Verification items for the finished model (mm, model axes). A direction names the side the tool comes from. Coordinates: 2 decimals unless noted, no trailing zeros. Loops run counter-clockwise (first coordinate to the right, second up) from the corner with the lowest first, then second, coordinate; pieces in that order, holes last. Notation, with made-up numbers: (8.5, -12.5) -> (32.5, -12.5) arc R6 cw to (32.5, -4.5) -> close; hole circle Ø11 at (69.5, -21.5). An arc over 180 degrees is marked (long way). Use CSV: the item, a comma, the result in double quotes. Start each with the question number.
```python
from build123d import *

# Parameters (mm, degrees)
F0_W     = 10
F0_H     = 10
F1_DEPTH = 5


with BuildPart() as f1:
    # F0 (on Top) → F1 (new body)
    with BuildSketch(Plane.XY):
        with BuildLine():
            Line((-217.772444, 298.14717), (-218.393043, 298.14717))
            Line((-218.393043, 298.14717), (-218.393043, 218.14717))
            Line((-218.393043, 218.14717), (-213.393043, 218.14717))
            Line((-213.393043, 218.14717), (-213.393043, 208.14717))
            Line((-213.393043, 208.14717), (-218.393043, 208.14717))
            Line((-218.393043, 208.14717), (-218.393043, 129.632429))
            ThreePointArc((-218.393043, 129.632429), (-108.393043, 172.033314), (1.606957, 129.632429))
            Line((1.606957, 129.632429), (1.606957, 208.14717))
            Line((1.606957, 208.14717), (-3.393043, 208.14717))
            Line((-3.393043, 208.14717), (-3.393043, 218.14717))
            Line((-3.393043, 218.14717), (1.606957, 218.14717))
            Line((1.606957, 218.14717), (1.606957, 298.14717))
            Line((1.606957, 298.14717), (0.986359, 298.14717))
            ThreePointArc((0.986359, 298.14717), (-108.393043, 255.777673), (-217.772444, 298.14717))
        make_face()
        with Locations((-203.393043, 213.14717)):
            Rectangle(F0_W, F0_H, mode=Mode.SUBTRACT)
        with Locations((-13.393043, 213.14717)):
            Rectangle(F0_W, F0_H, mode=Mode.SUBTRACT)
    extrude(amount=F1_DEPTH)


solid = f1.part
```
1. Depth check by flat-ended pin: pin 1 (3 mm diameter, centred on x = -54.5, z = 4.5, fed in from +Y); pin 2 (1.5 mm diameter, centred on x = -215, z = 2.5, fed in from -Y); pin 3 (1.5 mm diameter, centred on x = -216.5, z = 3, fed in from +Y). Enter the tip coordinate at first touch or a pass-through.
2. Cross-section at B-B, the plane y = 268. Record the boundary of the cut face in (x, z), plus the area to 3 significant figures.
3. Cross-section at D-D, the plane x = -126.5. Record the boundary of the cut face in (y, z).
4. Scan lines: line 1 (X direction, y = 213, z = 3.7); line 2 (X direction, y = 138, z = 4.75); line 3 (Y direction, x = -108.5, z = 2.4). Record each from-to range of solid material in increasing order.
5. Cross-section at A-A, the plane z = 0.9. Record the boundary of the cut face in (x, y), plus the area to 3 significant figures.
6. Cross-section at C-C, the plane x = -15. Record the boundary of the cut face in (y, z), plus the area to 3 significant figures.
7. Set-up check for faces 1 (the flat face through (-213.393, 213, 2)), 2 (the flat face through (-110, 215, 5)), 3 (the flat face through (-18.393, 213, 2)), 4 (the flat face through (-3.393, 213, 2)), 5 (the flat face through (1.607, 168, 2)): record each of +Z, -Z, +X, -X, +Y, -Y from which the full face is reachable in a straight line by a thin tool's end or side.
8. Release check for a two-part mould opening along Y. For faces 6 (the flat face through (-216, 218.147, 2)), 7 (the cylindrical face through (-106.713, 255.786, 2.465)), 8 (the flat face through (1.607, 258, 2)) record: released by +Y, released by -Y, zero draft, split by the parting line, or undercut.
Solution:
1,pin 1,"stops at y = 265.52"
1,pin 2,"stops at y = 131.97"
1,pin 3,"stops at y = 297.67"
2,outline,"(-218.39, 0) -> (-170.2, 0) -> (-170.2, 5) -> (-218.39, 5) -> close; (-46.59, 0) -> (1.61, 0) -> (1.61, 5) -> (-46.59, 5) -> close"
2,area,"482 mm2"
3,outline,"(171.03, 0) -> (256.79, 0) -> (256.79, 5) -> (171.03, 5) -> close"
4,line 1,"x = -213.39 to -208.39, -198.39 to -18.39, -8.39 to -3.39"
4,line 2,"x = -218.39 to -208.38, -8.41 to 1.61"
4,line 3,"y = 172.03 to 255.78"
5,outline,"(-218.39, 129.63) arc R163.89 cw to (1.61, 129.63) -> (1.61, 208.15) -> (-3.39, 208.15) -> (-3.39, 218.15) -> (1.61, 218.15) -> (1.61, 298.15) -> (0.99, 298.15) arc R162.37 cw to (-217.77, 298.15) -> (-218.39, 298.15) -> (-218.39, 218.15) -> (-213.39, 218.15) -> (-213.39, 208.15) -> (-218.39, 208.15) -> close; hole (-208.39, 208.15) -> (-198.39, 208.15) -> (-198.39, 218.15) -> (-208.39, 218.15) -> close; hole (-18.39, 208.15) -> (-8.39, 208.15) -> (-8.39, 218.15) -> (-18.39, 218.15) -> close"
5,area,"24,000 mm2"
6,outline,"(142.82, 0) -> (208.15, 0) -> (208.15, 5) -> (142.82, 5) -> close; (218.15, 0) -> (285.33, 0) -> (285.33, 5) -> (218.15, 5) -> close"
6,area,"663 mm2"
7,face 1,"+Z, -Z, -X"
7,face 2,"+Z, +X, -X, +Y, -Y"
7,face 3,"+Z, -Z"
7,face 4,"+Z, -Z, +X"
7,face 5,"+Z, -Z, +X, +Y, -Y"
8,face 6,"undercut"
8,face 7,"released by +Y"
8,face 8,"zero draft"
